```python
from build123d import *

# Parameters (mm, degrees)
F0_R     = 2.5
F1_DEPTH = 10
F2_SIZE  = 0.5
F3_R     = 4.25
F3_R_2   = 2.5
F4_DEPTH = 5
F6_DEPTH = 4
F7_R     = 0.3


with BuildPart() as f1:
    # F0 (on Front) → F1 (new body)
    with BuildSketch(Plane.XZ):
        Circle(F0_R)
    extrude(amount=F1_DEPTH)

    # F2
    f2_edges = [f1.edges().sort_by_distance(p)[0] for p in [
        (-2.5, -10, 0),
    ]]
    chamfer(f2_edges, length=F2_SIZE)

    # F3 (on face) → F4 (join)
    with BuildSketch(Plane(origin=(0, 0, 0), x_dir=(-1, 0, 0), z_dir=(0, 1, 0))):
        Circle(F3_R)
        Circle(F3_R_2, mode=Mode.SUBTRACT)
        Circle(F3_R_2)
    extrude(amount=F4_DEPTH)

    # F5 (on face) → F6 (cut)
    with BuildSketch(Plane(origin=(0, 5, 0), x_dir=(-1, 0, 0), z_dir=(0, 1, 0))):
        Polygon((-0.2009555222, 2.3006412609), (-2.092891538, 0.9762880432), (-1.8919360159, -1.3243532177), (0.2009555222, -2.3006412609), (2.092891538, -0.9762880432), (1.8919360159, 1.3243532177), align=None)
    extrude(amount=-F6_DEPTH, mode=Mode.SUBTRACT)

    # F7
    f7_edges = [f1.edges().sort_by_distance(p)[0] for p in [
        (4.25, 5, 0),
        (4.25, 0, 0),
        (1.146924, 5, 1.638465),
        (-0.84549, 5, 1.812497),
        (1.992414, 5, -0.174033),
        (0.84549, 5, -1.812497),
        (-1.146924, 5, -1.638465),
        (-1.992414, 5, 0.174033),
    ]]
    fillet(f7_edges, radius=F7_R)


solid = f1.part
```
Geometry: final body of the model. Coordinates: model frame, mm. A direction names the side the tool comes from. Coordinates: 2 decimals unless noted, no trailing zeros. Order: outer loops, then holes, each group sorted by start corner. A loop starts at its lowest first (then second) coordinate and runs counter-clockwise, first axis right, second up. Notation, with made-up numbers: (-22, -34) -> (-11, -34) arc R30 cw to (-11, -3) -> close; hole circle Ø5 at (89.5, 15.25). An arc over 180 degrees is marked (long way). Write each question's results on one line, items separated by ' | '. Start each with the question number.
1) Material intervals for line 1 along Z through (x, y) = (-0.5, 3.5); line 2 along Y through (x, z) = (1.5, -1.25); line 3 along Y through (x, z) = (3.25, 0), sorted ascending.
2) First-contact query: pin 1 (2 mm diameter, centred on x = -1, y = -5, fed in from +Z); pin 2 (1.3 mm diameter, centred on x = -0.5, z = -0.5, fed in from +Y); pin 3 (2 mm diameter, centred on y = -2, z = -3, fed in from +X). Flat tips, straight axial feed; report the tip coordinate or a pass-through.
3) Cut plane B-B, the plane y = -7. Output: boundary loops of the cut face in (x, z), and give its area (3 significant figures).
4) Mould query, pull axis X, two halves, no side actions, for faces 4 (the cylindrical face through (-2.285, 2.469, 3.584)), 5 (the flat face through (0.86, 2.876, -1.806)), 6 (the flat face through (0, 0, -3)). Classes: released by +X, released by -X, zero draft, split by the parting line, or undercut.
5) Set-up query: faces 1 (the flat face through (-2, 5, -2)), 2 (the cylindrical face through (-0.54, -4.68, -2.44)), 3 (the flat face through (1.994, 2.876, -0.158)). Return all of +Z, -Z, +X, -X, +Y, -Y with unobstructed straight access to the full face (end or side cutting, diameter ignored); none if empty.
6) Cut plane A-A, the plane y = 3.5. Output: boundary loops of the cut face in (x, z).
7) Cut plane C-C, the plane y = 0.5. Output: boundary loops of the cut face in (x, z), and give its area (3 significant figures).
Checks:
1) line 1: -4.22 to -2.09, 1.97 to 4.22 | line 2: -10 to 1 | line 3: 0 to 5
2) pin 1: z = 2.5 | pin 2: y = 1 | pin 3: x = 1.5
3) outline: circle Ø5 at (0, 0) | area: 19.6 mm^2
4) face 4: split by the parting line | face 5: undercut | face 6: zero draft
5) face 1: +Z, -Z, +X, -X, +Y | face 2: -Y | face 3: +Y
6) outline: circle Ø8.5 at (0, 0); hole (-2.09, -0.98) -> (-0.2, -2.3) -> (1.89, -1.32) -> (2.09, 0.98) -> (0.2, 2.3) -> (-1.89, 1.32) -> close
7) outline: circle Ø8.5 at (0, 0) | area: 56.7 mm^2
